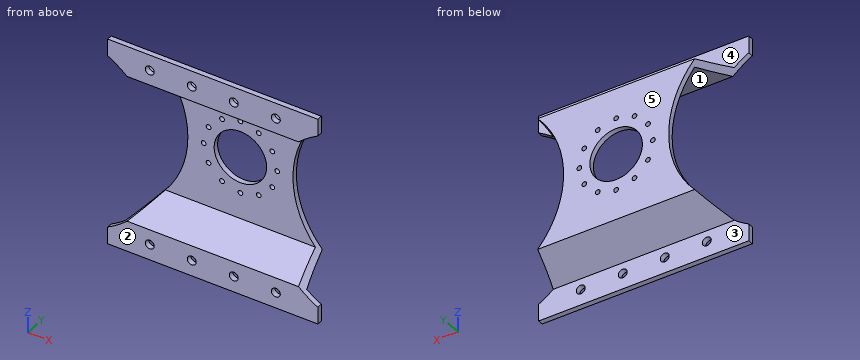
from build123d import *

# Parameters (mm, degrees)
EXTRUDE_1_DEPTH     = 200
SKETCH_2_R          = 95
CUT_EXTRUDE_1_DEPTH = 150
SKETCH_3_R          = 4.25
CUT_EXTRUDE_2_DEPTH = 150
SKETCH_4_R          = 2.25
SKETCH_4_R_2        = 25
CUT_EXTRUDE_3_DEPTH = 10


with BuildPart() as part:
    # 草图1 → 凸台-拉伸1 (new body)
    with BuildSketch(Plane(origin=(0, 0, 0), x_dir=(0, 0, -1), z_dir=(1, 0, 0))):
        Polygon((-100, 0), (-70.717967697, 0), (-60, 40), (60, 40), (70.717967697, 0), (100, 0), (100, 5), (74.554602637, 5), (63.83663494, 45), (-63.83663494, 45), (-74.554602637, 5), (-100, 5), align=None)
    extrude(amount=EXTRUDE_1_DEPTH)

    # 草图2 → 切除-拉伸1 (cut)
    with BuildSketch(Plane(origin=(0, 45, 0), x_dir=(1, 0, 0), z_dir=(0, 1, 0))):
        with Locations((245, 0)):
            Circle(SKETCH_2_R)
        with Locations((-45, 0)):
            Circle(SKETCH_2_R)
    extrude(amount=-CUT_EXTRUDE_1_DEPTH, mode=Mode.SUBTRACT)

    # 草图3 → 切除-拉伸2 (cut)
    with BuildSketch(Plane(origin=(0, 5, 0), x_dir=(1, 0, 0), z_dir=(0, 1, 0))):
        with Locations(Location((120, -85, 0), (0, 0, 270))):
            Circle(SKETCH_3_R)
        with Locations(Location((160, -85, 0), (0, 0, 270))):
            Circle(SKETCH_3_R)
        with Locations(Location((40, -85, 0), (0, 0, 270))):
            Circle(SKETCH_3_R)
        with Locations(Location((80, -85, 0), (0, 0, 270))):
            Circle(SKETCH_3_R)
        with Locations(Location((160, 85, 0), (0, 0, 270))):
            Circle(SKETCH_3_R)
        with Locations(Location((120, 85, 0), (0, 0, 270))):
            Circle(SKETCH_3_R)
        with Locations(Location((80, 85, 0), (0, 0, 270))):
            Circle(SKETCH_3_R)
        with Locations(Location((40, 85, 0), (0, 0, 270))):
            Circle(SKETCH_3_R)
    extrude(amount=-CUT_EXTRUDE_2_DEPTH, mode=Mode.SUBTRACT)

    # 草图4 → 切除-拉伸3 (cut)
    with BuildSketch(Plane(origin=(0, 45, 0), x_dir=(1, 0, 0), z_dir=(0, 1, 0))):
        with Locations(Location((100, 35, 0), (0, 0, 270))):
            Circle(SKETCH_4_R)
        with Locations(Location((117.5, 30.310889132, 0), (0, 0, 270))):
            Circle(SKETCH_4_R)
        with Locations(Location((130.310889132, 17.5, 0), (0, 0, 270))):
            Circle(SKETCH_4_R)
        with Locations(Location((135, 0, 0), (0, 0, 270))):
            Circle(SKETCH_4_R)
        with Locations(Location((130.310889132, -17.5, 0), (0, 0, 270))):
            Circle(SKETCH_4_R)
        with Locations(Location((117.5, -30.310889132, 0), (0, 0, 270))):
            Circle(SKETCH_4_R)
        with Locations(Location((100, -35, 0), (0, 0, 270))):
            Circle(SKETCH_4_R)
        with Locations(Location((82.5, -30.310889132, 0), (0, 0, 270))):
            Circle(SKETCH_4_R)
        with Locations(Location((69.689110868, -17.5, 0), (0, 0, 270))):
            Circle(SKETCH_4_R)
        with Locations(Location((65, 0, 0), (0, 0, 270))):
            Circle(SKETCH_4_R)
        with Locations(Location((69.689110868, 17.5, 0), (0, 0, 270))):
            Circle(SKETCH_4_R)
        with Locations(Location((82.5, 30.310889132, 0), (0, 0, 270))):
            Circle(SKETCH_4_R)
        with Locations(Location((100, 0, 0), (0, 0, 270))):
            Circle(SKETCH_4_R_2)
    extrude(amount=-CUT_EXTRUDE_3_DEPTH, mode=Mode.SUBTRACT)


solid = part.part
Could you check a few things on this model? Use its own coordinates, in mm. Face numbers are marked on the shaded views. A direction names the side the tool comes from. Coordinates: 2 decimals unless noted, no trailing zeros. Write each loop counter-clockwise with the first axis right and the second up, starting at its lowest first coordinate (ties: lowest second). Pieces come first, ordered by that corner, then holes. Notation, with made-up numbers: (10.5, 70) - (63.5, 70) arc R32 cw to (63.5, 109) - close; hole circle Ø1 at (70, 30). An arc over 180 degrees is marked (long way). Put each result on its own line as item: value. Start each with the question number.
Q1. I'm going to push flat-ended pins straight in: P1, Ø7, axis at x = 69.69, z = -17.5, coming from the +Y side; P2, Ø6, axis at y = 10.5, z = 71.5, coming from the +X side; P3, Ø5, axis at x = 117.5, z = -30.31, coming from the -Y side; P4, Ø10, axis at x = 80, z = -85, coming from the +Y side. Where does each tip first touch, or does it pass through?
Q2. I want a section at A-A on x = 168. Write out the boundary of the cut face in (y, z).
Q3. Which directions (+Z, -Z, +X, -X, +Y, -Y) give clear straight access to the entire face, cutting with the end or side of a thin tool? Please do the marked faces 1, 2, 3, 4 and 5.
Q4. Please list where these lines run through material, in increasing order: L1, parallel to X at y = 2, z = 85; L2, parallel to X at y = 42.5, z = 0; L3, parallel to Y at x = 103, z = -38.
Checks:
1. P1: y = 45
1. P2: x = 184.99
1. P3: y = 40
1. P4: y = 5
2. outline: (0, -100) - (5, -100) - (5, -74.55) - (45, -63.84) - (45, -55.64) - (40, -55.64) - (40, -60) - (0, -70.72) - close; (0, 70.72) - (40, 60) - (40, 55.64) - (45, 55.64) - (45, 63.84) - (5, 74.55) - (5, 100) - (0, 100) - close
3. face 1: +X, -X, -Y
3. face 2: +Z, -Z, +X, -X, -Y
3. face 3: -Z, +X, -X, +Y
3. face 4: +Z, +X, -X, +Y
3. face 5: +Z, -Z, +X, -X, +Y
4. L1: 0 to 35.75, 44.25 to 75.75, 84.25 to 115.75, 124.25 to 155.75, 164.25 to 200
4. L2: 50 to 62.75, 67.25 to 75, 125 to 132.75, 137.25 to 150
4. L3: 40 to 45
